```python
from build123d import *

# Parameters (mm, degrees)
F1_DEPTH = 6.35


with BuildPart() as f1:
    # F0 (on Top) → F1 (new body)
    with BuildSketch(Plane.XY):
        with BuildLine():
            ThreePointArc((-98.5, -52.65), (-96.640128, -57.140128), (-92.15, -59))
            Line((-92.15, -59), (-19.05, -59))
            ThreePointArc((-19.05, -59), (-5.579616, -64.579616), (0, -78.05))
            Line((0, -78.05), (0, -80.95))
            ThreePointArc((0, -80.95), (5.579616, -94.420384), (19.05, -100))
            Line((19.05, -100), (86.15, -100))
            ThreePointArc((86.15, -100), (90.640128, -98.140128), (92.5, -93.65))
            Line((92.5, -93.65), (92.5, -63.117434))
            ThreePointArc((92.5, -63.117434), (91.877326, -60.375129), (90.131422, -58.170639))
            ThreePointArc((90.131422, -58.170639), (62.278704, 0), (90.131422, 58.170639))
            ThreePointArc((90.131422, 58.170639), (91.877326, 60.375129), (92.5, 63.117434))
            Line((92.5, 63.117434), (92.5, 93.65))
            ThreePointArc((92.5, 93.65), (90.640128, 98.140128), (86.15, 100))
            Line((86.15, 100), (15.45, 100))
            ThreePointArc((15.45, 100), (1.979616, 94.420384), (-3.6, 80.95))
            Line((-3.6, 80.95), (-3.6, 76))
            Line((-3.6, 76), (-3.6, 47.35))
            ThreePointArc((-3.6, 47.35), (-5.459872, 42.859872), (-9.95, 41))
            Line((-9.95, 41), (-35.35, 41))
            ThreePointArc((-35.35, 41), (-39.840128, 42.859872), (-41.7, 47.35))
            Line((-41.7, 47.35), (-41.7, 69.65))
            ThreePointArc((-41.7, 69.65), (-43.559872, 74.140128), (-48.05, 76))
            Line((-48.05, 76), (-92.15, 76))
            ThreePointArc((-92.15, 76), (-96.640128, 74.140128), (-98.5, 69.65))
            Line((-98.5, 69.65), (-98.5, 51.389104))
            ThreePointArc((-98.5, 51.389104), (-97.119749, 47.436371), (-93.579024, 45.201989))
            ThreePointArc((-93.579024, 45.201989), (-64.387776, 8.5), (-93.579024, -28.201989))
            ThreePointArc((-93.579024, -28.201989), (-97.119749, -30.436371), (-98.5, -34.389104))
            Line((-98.5, -34.389104), (-98.5, -52.65))
        make_face()
    extrude(amount=-F1_DEPTH)


solid = f1.part
```
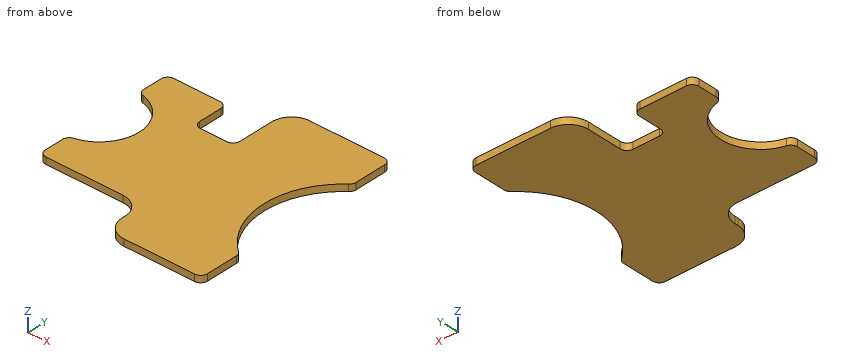
Can you work these out from the model? Positions are in its coordinate system, mm. Coordinates: 2 decimals unless noted, no trailing zeros. Loops run counter-clockwise (first coordinate to the right, second up) from the corner with the lowest first, then second, coordinate; pieces in that order, holes last. Notation, with made-up numbers: (-38, 60) -> (10, 60) arc R22 ccw to (10, 91) -> close; hole circle Ø6 at (-16, 1.25). An arc over 180 degrees is marked (long way). Answer as a JSON object with one key per item and string values.
1) Imagine slicing it at B-B (y = 60.5). Please give me the cut outline in (x, z), then the cut area to 3 significant figures.
Results:
{"outline": "(-98.5, -6.35) -> (-41.7, -6.35) -> (-41.7, 0) -> (-98.5, 0) -> close; (-3.6, -6.35) -> (91.94, -6.35) -> (91.94, 0) -> (-3.6, 0) -> close", "area": "967 mm^2"}
2) Imagine slicing it at A-A (x = -70.5). Please give me the cut outline in (y, z).
Results:
{"outline": "(-59, -6.35) -> (-12.07, -6.35) -> (-12.07, 0) -> (-59, 0) -> close; (29.07, -6.35) -> (76, -6.35) -> (76, 0) -> (29.07, 0) -> close"}
3) If I drill on line 1 (X direction, y = 82, z = -1.25); line 2 (X direction, y = 60, z = -5.75); line 3 (Y direction, x = -83.5, z = -1), over which ranges is the centre line in solid material (lowest first)?
Results:
{"line 1": "x = -3.57 to 92.5", "line 2": "x = -98.5 to -41.7, -3.6 to 91.68", "line 3": "y = -59 to -24.28, 41.28 to 76"}
4) Imagine slicing it at D-D (x = -39). Please give me the cut outline in (y, z).
Results:
{"outline": "(-59, -6.35) -> (42.15, -6.35) -> (42.15, 0) -> (-59, 0) -> close"}
5) Imagine slicing it at C-C (z = -1). Please give me the cut outline in (x, y), then the cut area to 3 significant figures.
Results:
{"outline": "(-98.5, -52.65) arc R6.35 ccw to (-92.15, -59) -> (-19.05, -59) arc R19.05 cw to (0, -78.05) -> (0, -80.95) arc R19.05 ccw to (19.05, -100) -> (86.15, -100) arc R6.35 ccw to (92.5, -93.65) -> (92.5, -63.12) arc R6.35 ccw to (90.13, -58.17) arc R74.67 cw to (90.13, 58.17) arc R6.35 ccw to (92.5, 63.12) -> (92.5, 93.65) arc R6.35 ccw to (86.15, 100) -> (15.45, 100) arc R19.05 ccw to (-3.6, 80.95) -> (-3.6, 47.35) arc R6.35 cw to (-9.95, 41) -> (-35.35, 41) arc R6.35 cw to (-41.7, 47.35) -> (-41.7, 69.65) arc R6.35 ccw to (-48.05, 76) -> (-92.15, 76) arc R6.35 ccw to (-98.5, 69.65) -> (-98.5, 51.39) arc R6.35 ccw to (-93.58, 45.2) arc R37.67 cw to (-93.58, -28.2) arc R6.35 ccw to (-98.5, -34.39) -> close", "area": "25,900 mm^2"}
6) For P1, Ø3, axis at y = 18, z = -4.5, coming from the +X side; P2, Ø2, axis at x = -61, z = -5.5, coming from the +Y side; P3, Ø12, axis at x = 61, y = 31.5, coming from the +Z side; P4, Ø2.5, axis at y = -80, z = -3.5, coming from the -X side, each with a flat end and sliding along its axis, tell me the tip position at first contact or that it passes through.
Results:
{"P1": "stops at x = 64.87", "P2": "stops at y = 76", "P3": "stops at z = 0", "P4": "stops at x = 0"}
